```python
from build123d import *

# Parameters (mm, degrees)
SKETCH1_R           = 4
BOSS_EXTRUDE1_DEPTH = 16
SKETCH2_R           = 3
BOSS_EXTRUDE2_DEPTH = 15
SKETCH3_R           = 1.25
CUT_EXTRUDE1_DEPTH  = 40
CHAMFER1_SIZE       = 0.5


with BuildPart() as part:
    # Sketch1 → Boss-Extrude1 (new body)
    with BuildSketch(Plane.XY):
        with Locations((-161.229707574, -61.073300905)):
            Circle(SKETCH1_R)
    extrude(amount=BOSS_EXTRUDE1_DEPTH)

    # Sketch2 → Boss-Extrude2 (add)
    with BuildSketch(Plane.XY.offset(16)):
        with Locations((-161.229707574, -61.073300905)):
            Circle(SKETCH2_R)
    extrude(amount=BOSS_EXTRUDE2_DEPTH)

    # Sketch3 → Cut-Extrude1 (cut)
    with BuildSketch(Plane.XY.offset(31)):
        with Locations((-161.229707574, -61.073300905)):
            Circle(SKETCH3_R)
    extrude(amount=-CUT_EXTRUDE1_DEPTH, mode=Mode.SUBTRACT)

    # Chamfer1
    chamfer1_edges = [part.edges().sort_by_distance(p)[0] for p in [
        (-165.229707574, -61.073300905, 0),
        (-164.229707574, -61.073300905, 31),
    ]]
    chamfer(chamfer1_edges, length=CHAMFER1_SIZE)


solid = part.part
```
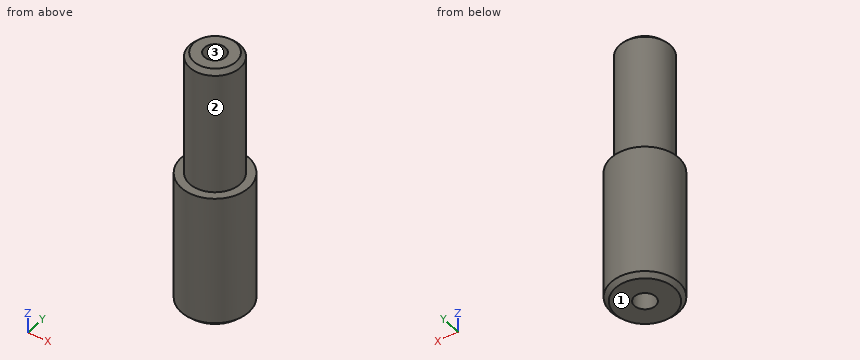
For this review, take the finished solid that the model builds, in its own axes (mm). Face numbers are marked on the shaded views. Round coordinates to 2 decimals unless told otherwise and drop trailing zeros. Order: outer loops, then holes, each group sorted by start corner. A loop starts at its lowest first (then second) coordinate and runs counter-clockwise, first axis right, second up.
Q1. We need section A-A, the plane z = 5. Give the boundary of the cut face in (x, y).
Findings below:
outline: circle Ø8 at (-161.23, -61.07); hole circle Ø2.5 at (-161.23, -61.07)
Q2. Mouldability with a two-part tool opening along Y and no side actions: class the marked faces 1, 2 and 3 as pulls with the +Y half, pulls with the -Y half, needs draft (parallel to the pull), parting line crosses it, or undercut.
Findings below:
face 1: needs draft
face 2: parting line crosses it
face 3: undercut
Q3. We need section B-B, the plane z = 24.5. Give the boundary of the cut face in (x, y), plus the area to 3 significant figures.
Findings below:
outline: circle Ø6 at (-161.23, -61.07); hole circle Ø2.5 at (-161.23, -61.07)
area: 23.4 mm2
Q4. Wall thickness on line 1 (Z direction, x = -161.75, y = -64.5); line 2 (X direction, y = -63, z = 13.5); line 3 (X direction, y = -61.75, z = 28.5): over which ranges is each line inside the solid? List them lowest first.
Findings below:
line 1: z = 0 to 16
line 2: x = -164.74 to -157.72
line 3: x = -164.15 to -162.28, -160.18 to -158.31
Q5. Insertion check: P1, Ø1.5, axis at y = -63, z = 16, coming from the -X side; P2, Ø1, axis at x = -164.5, z = 19.5, coming from the +Y side; P3, Ø3, axis at y = -62.5, z = 23.5, coming from the -X side; P4, Ø1.5, axis at x = -161.23, y = -61.07, coming from the +Z side. Each pin has a flat end and moves straight along its axis. Give the tip position at first contact, or say it passes through.
Findings below:
P1: stops at x = -165.05
P2: stops at y = -59.92
P3: stops at x = -164.23
P4: passes through
